Geometry check sheet. Reference: the model listing, model coordinates, mm. A direction names the side the tool comes from. Round coordinates to 2 decimals unless told otherwise and drop trailing zeros. Write each loop counter-clockwise with the first axis right and the second up, starting at its lowest first coordinate (ties: lowest second). Pieces come first, ordered by that corner, then holes. Notation, with made-up numbers: (-29, -29.5) -> (-7, -29.5) arc R33 cw to (-7, 7.5) -> close; hole circle Ø10 at (77.5, 42.5). An arc over 180 degrees is marked (long way). One line per question, with ' | ' between items.
```python
from build123d import *

# Parameters (mm, degrees)
SKETCH1_R           = 1.600003175
SKETCH1_W           = 1.5
SKETCH1_H           = 42.00008382
SKETCH1_W_2         = 92.00018542
SKETCH1_H_2         = 1.5
BOSS_EXTRUDE1_DEPTH = 3
SKETCH1_3_W         = 92.00018542
SKETCH1_3_H         = 1.5
SKETCH1_3_W_2       = 1.5
SKETCH1_3_H_2       = 42.00008382
BOSS_EXTRUDE2_DEPTH = 16


with BuildPart() as part:
    # Sketch1 → Boss-Extrude1 (new body)
    # profile 1 of 17: a face of its own
    with BuildSketch(Plane(origin=(0, 0, 0), x_dir=(1, 0, 0), z_dir=(0, 1, 0))):
        with BuildLine():
            Line((96.00019304, 49.987399035), (4.00000762, 49.987399035))
            ThreePointArc((4.00000762, 49.987399035), (1.180555381, 48.819543679), (0.012700025, 46.00009144))
            Line((0.012700025, 46.00009144), (0.012700025, 4.00000762))
            ThreePointArc((0.012700025, 4.00000762), (1.180555381, 1.180555381), (4.00000762, 0.012700025))
            Line((4.00000762, 0.012700025), (96.00019304, 0.012700025))
            ThreePointArc((96.00019304, 0.012700025), (98.819645279, 1.180555381), (99.987500635, 4.00000762))
            Line((99.987500635, 4.00000762), (99.987500635, 46.00009144))
            ThreePointArc((99.987500635, 46.00009144), (98.819645279, 48.819543679), (96.00019304, 49.987399035))
        make_face()
        with Locations(Location((5.00001016, 45.0000889, 0), (0, 0, 270))):
            Circle(SKETCH1_R, mode=Mode.SUBTRACT)
        with Locations(Location((5.00001016, 5.00001016, 0), (0, 0, 270))):
            Circle(SKETCH1_R, mode=Mode.SUBTRACT)
        with Locations(Location((95.0001905, 5.00001016, 0), (0, 0, 270))):
            Circle(SKETCH1_R, mode=Mode.SUBTRACT)
        with Locations(Location((95.0001905, 45.0000889, 0), (0, 0, 270))):
            Circle(SKETCH1_R, mode=Mode.SUBTRACT)
        with BuildLine():
            Line((85.627156504, 17.327051436), (70.827156816, 17.327051436))
            ThreePointArc((70.827156816, 17.327051436), (70.473603433, 17.473498042), (70.327156827, 17.827051425))
            Line((70.327156827, 17.827051425), (70.327156827, 36.027051041))
            ThreePointArc((70.327156827, 36.027051041), (70.473603433, 36.380604424), (70.827156816, 36.52705103))
            Line((70.827156816, 36.52705103), (85.627156504, 36.52705103))
            ThreePointArc((85.627156504, 36.52705103), (85.980709887, 36.380604424), (86.127156493, 36.027051041))
            Line((86.127156493, 36.027051041), (86.127156493, 17.827051425))
            ThreePointArc((86.127156493, 17.827051425), (85.980709887, 17.473498042), (85.627156504, 17.327051436))
        make_face(mode=Mode.SUBTRACT)
    # profile 2 of 17: a face of its own
    with BuildSketch(Plane(origin=(0, 0, 0), x_dir=(1, 0, 0), z_dir=(0, 1, 0))):
        with Locations((-0.737299975, 25.00004953)):
            Rectangle(SKETCH1_W, SKETCH1_H)
    # profile 3 of 17: a face of its own
    with BuildSketch(Plane(origin=(0, 0, 0), x_dir=(1, 0, 0), z_dir=(0, 1, 0))):
        with Locations((-2.237299975, 25.00004953)):
            Rectangle(SKETCH1_W, SKETCH1_H)
    # profile 4 of 17: a face of its own
    with BuildSketch(Plane(origin=(0, 0, 0), x_dir=(1, 0, 0), z_dir=(0, 1, 0))):
        with BuildLine():
            ThreePointArc((4.00000762, -1.487299975), (0.119895209, 0.119895209), (-1.487299975, 4.00000762))
            Line((-1.487299975, 4.00000762), (-2.987299975, 4.00000762))
            ThreePointArc((-2.987299975, 4.00000762), (-0.940764962, -0.940764962), (4.00000762, -2.987299975))
            Line((4.00000762, -2.987299975), (4.00000762, -1.487299975))
        make_face()
    # profile 5 of 17: a face of its own
    with BuildSketch(Plane(origin=(0, 0, 0), x_dir=(1, 0, 0), z_dir=(0, 1, 0))):
        with BuildLine():
            ThreePointArc((4.00000762, 0.012700025), (1.180555381, 1.180555381), (0.012700025, 4.00000762))
            Line((0.012700025, 4.00000762), (-1.487299975, 4.00000762))
            ThreePointArc((-1.487299975, 4.00000762), (0.119895209, 0.119895209), (4.00000762, -1.487299975))
            Line((4.00000762, -1.487299975), (4.00000762, 0.012700025))
        make_face()
    # profile 6 of 17: a face of its own
    with BuildSketch(Plane(origin=(0, 0, 0), x_dir=(1, 0, 0), z_dir=(0, 1, 0))):
        with Locations((50.00010033, -0.737299975)):
            Rectangle(SKETCH1_W_2, SKETCH1_H_2)
    # profile 7 of 17: a face of its own
    with BuildSketch(Plane(origin=(0, 0, 0), x_dir=(1, 0, 0), z_dir=(0, 1, 0))):
        with Locations((50.00010033, -2.237299975)):
            Rectangle(SKETCH1_W_2, SKETCH1_H_2)
    # profile 8 of 17: a face of its own
    with BuildSketch(Plane(origin=(0, 0, 0), x_dir=(1, 0, 0), z_dir=(0, 1, 0))):
        with BuildLine():
            Line((101.487500635, 4.00000762), (99.987500635, 4.00000762))
            ThreePointArc((99.987500635, 4.00000762), (98.819645279, 1.180555381), (96.00019304, 0.012700025))
            Line((96.00019304, 0.012700025), (96.00019304, -1.487299975))
            ThreePointArc((96.00019304, -1.487299975), (99.880305451, 0.119895209), (101.487500635, 4.00000762))
        make_face()
    # profile 9 of 17: a face of its own
    with BuildSketch(Plane(origin=(0, 0, 0), x_dir=(1, 0, 0), z_dir=(0, 1, 0))):
        with BuildLine():
            Line((102.987500635, 4.00000762), (101.487500635, 4.00000762))
            ThreePointArc((101.487500635, 4.00000762), (99.880305451, 0.119895209), (96.00019304, -1.487299975))
            Line((96.00019304, -1.487299975), (96.00019304, -2.987299975))
            ThreePointArc((96.00019304, -2.987299975), (100.940965623, -0.940764962), (102.987500635, 4.00000762))
        make_face()
    # profile 10 of 17: a face of its own
    with BuildSketch(Plane(origin=(0, 0, 0), x_dir=(1, 0, 0), z_dir=(0, 1, 0))):
        with Locations((100.737500635, 25.00004953)):
            Rectangle(SKETCH1_W, SKETCH1_H)
    # profile 11 of 17: a face of its own
    with BuildSketch(Plane(origin=(0, 0, 0), x_dir=(1, 0, 0), z_dir=(0, 1, 0))):
        with Locations((102.237500635, 25.00004953)):
            Rectangle(SKETCH1_W, SKETCH1_H)
    # profile 12 of 17: a face of its own
    with BuildSketch(Plane(origin=(0, 0, 0), x_dir=(1, 0, 0), z_dir=(0, 1, 0))):
        with BuildLine():
            Line((96.00019304, 51.487399035), (96.00019304, 49.987399035))
            ThreePointArc((96.00019304, 49.987399035), (98.819645279, 48.819543679), (99.987500635, 46.00009144))
            Line((99.987500635, 46.00009144), (101.487500635, 46.00009144))
            ThreePointArc((101.487500635, 46.00009144), (99.880305451, 49.880203851), (96.00019304, 51.487399035))
        make_face()
    # profile 13 of 17: a face of its own
    with BuildSketch(Plane(origin=(0, 0, 0), x_dir=(1, 0, 0), z_dir=(0, 1, 0))):
        with BuildLine():
            Line((96.00019304, 52.987399035), (96.00019304, 51.487399035))
            ThreePointArc((96.00019304, 51.487399035), (99.880305451, 49.880203851), (101.487500635, 46.00009144))
            Line((101.487500635, 46.00009144), (102.987500635, 46.00009144))
            ThreePointArc((102.987500635, 46.00009144), (100.940965623, 50.940864023), (96.00019304, 52.987399035))
        make_face()
    # profile 14 of 17: a face of its own
    with BuildSketch(Plane(origin=(0, 0, 0), x_dir=(1, 0, 0), z_dir=(0, 1, 0))):
        with Locations((50.00010033, 50.737399035)):
            Rectangle(SKETCH1_W_2, SKETCH1_H_2)
    # profile 15 of 17: a face of its own
    with BuildSketch(Plane(origin=(0, 0, 0), x_dir=(1, 0, 0), z_dir=(0, 1, 0))):
        with Locations((50.00010033, 52.237399035)):
            Rectangle(SKETCH1_W_2, SKETCH1_H_2)
    # profile 16 of 17: a face of its own
    with BuildSketch(Plane(origin=(0, 0, 0), x_dir=(1, 0, 0), z_dir=(0, 1, 0))):
        with BuildLine():
            ThreePointArc((0.012700025, 46.00009144), (1.180555381, 48.819543679), (4.00000762, 49.987399035))
            Line((4.00000762, 49.987399035), (4.00000762, 51.487399035))
            ThreePointArc((4.00000762, 51.487399035), (0.119895209, 49.880203851), (-1.487299975, 46.00009144))
            Line((-1.487299975, 46.00009144), (0.012700025, 46.00009144))
        make_face()
    # profile 17 of 17: a face of its own
    with BuildSketch(Plane(origin=(0, 0, 0), x_dir=(1, 0, 0), z_dir=(0, 1, 0))):
        with BuildLine():
            ThreePointArc((-1.487299975, 46.00009144), (0.119895209, 49.880203851), (4.00000762, 51.487399035))
            Line((4.00000762, 51.487399035), (4.00000762, 52.987399035))
            ThreePointArc((4.00000762, 52.987399035), (-0.940764962, 50.940864023), (-2.987299975, 46.00009144))
            Line((-2.987299975, 46.00009144), (-1.487299975, 46.00009144))
        make_face()
    extrude(amount=BOSS_EXTRUDE1_DEPTH)

    # Sketch1_3 → Boss-Extrude2 (add)
    with BuildSketch(Plane(origin=(0, 0, 0), x_dir=(1, 0, 0), z_dir=(0, 1, 0))):
        with BuildLine():
            ThreePointArc((-1.487299975, 46.00009144), (0.119895209, 49.880203851), (4.00000762, 51.487399035))
            Line((4.00000762, 51.487399035), (4.00000762, 52.987399035))
            ThreePointArc((4.00000762, 52.987399035), (-0.940764962, 50.940864023), (-2.987299975, 46.00009144))
            Line((-2.987299975, 46.00009144), (-1.487299975, 46.00009144))
        make_face()
        with Locations((50.00010033, 52.237399035)):
            Rectangle(SKETCH1_3_W, SKETCH1_3_H)
        with BuildLine():
            Line((96.00019304, 52.987399035), (96.00019304, 51.487399035))
            ThreePointArc((96.00019304, 51.487399035), (99.880305451, 49.880203851), (101.487500635, 46.00009144))
            Line((101.487500635, 46.00009144), (102.987500635, 46.00009144))
            ThreePointArc((102.987500635, 46.00009144), (100.940965623, 50.940864023), (96.00019304, 52.987399035))
        make_face()
        with Locations((102.237500635, 25.00004953)):
            Rectangle(SKETCH1_3_W_2, SKETCH1_3_H_2)
        with BuildLine():
            Line((102.987500635, 4.00000762), (101.487500635, 4.00000762))
            ThreePointArc((101.487500635, 4.00000762), (99.880305451, 0.119895209), (96.00019304, -1.487299975))
            Line((96.00019304, -1.487299975), (96.00019304, -2.987299975))
            ThreePointArc((96.00019304, -2.987299975), (100.940965623, -0.940764962), (102.987500635, 4.00000762))
        make_face()
        with Locations((50.00010033, -2.237299975)):
            Rectangle(SKETCH1_3_W, SKETCH1_3_H)
        with BuildLine():
            ThreePointArc((4.00000762, -1.487299975), (0.119895209, 0.119895209), (-1.487299975, 4.00000762))
            Line((-1.487299975, 4.00000762), (-2.987299975, 4.00000762))
            ThreePointArc((-2.987299975, 4.00000762), (-0.940764962, -0.940764962), (4.00000762, -2.987299975))
            Line((4.00000762, -2.987299975), (4.00000762, -1.487299975))
        make_face()
        with Locations((-2.237299975, 25.00004953)):
            Rectangle(SKETCH1_3_W_2, SKETCH1_3_H_2)
    extrude(amount=BOSS_EXTRUDE2_DEPTH)


solid = part.part
```
(1) Draft check along X on faces 1 (the cylindrical face through (5.07, 1.48, -46.6)), 2 (the cylindrical face through (100.89, 7.89, 0.99)), 3 (the cylindrical face through (-0.89, 7.89, -50.99)). Enter one of: +X half, -X half, draft (parallel to the pull), parting line (faces both ways), or undercut.
Resolved:
face 1: undercut | face 2: +X half | face 3: -X half
(2) Sectioned sample at D-D on y = 15. Record the cut outline in (x, z), then the cut area to 3 significant figures.
Resolved:
outline: (-2.99, -46) arc R6.99 ccw to (4, -52.99) -> (96, -52.99) arc R6.99 ccw to (102.99, -46) -> (102.99, -4) arc R6.99 ccw to (96, 2.99) -> (4, 2.99) arc R6.99 ccw to (-2.99, -4) -> close; hole (-1.49, -46) arc R5.49 ccw to (4, -51.49) -> (96, -51.49) arc R5.49 ccw to (101.49, -46) -> (101.49, -4) arc R5.49 ccw to (96, 1.49) -> (4, 1.49) arc R5.49 ccw to (-1.49, -4) -> close | area: 461 mm2
(3) Sectioned sample at C-C on y = 1.25. Record the cut outline in (x, z).
Resolved:
outline: (-2.99, -46) arc R6.99 ccw to (4, -52.99) -> (96, -52.99) arc R6.99 ccw to (102.99, -46) -> (102.99, -4) arc R6.99 ccw to (96, 2.99) -> (4, 2.99) arc R6.99 ccw to (-2.99, -4) -> close; hole circle Ø3.2 at (5, -45); hole circle Ø3.2 at (5, -5); hole (70.33, -36.03) arc R0.5 ccw to (70.83, -36.53) -> (85.63, -36.53) arc R0.5 ccw to (86.13, -36.03) -> (86.13, -17.83) arc R0.5 ccw to (85.63, -17.33) -> (70.83, -17.33) arc R0.5 ccw to (70.33, -17.83) -> close; hole circle Ø3.2 at (95, -45); hole circle Ø3.2 at (95, -5)
(4) Sectioned sample at A-A on z = -19. Record the cut outline in (x, y), then the cut area to 3 significant figures.
Resolved:
outline: (-2.99, 0) -> (70.33, 0) -> (70.33, 3) -> (-1.49, 3) -> (-1.49, 16) -> (-2.99, 16) -> close; (86.13, 0) -> (102.99, 0) -> (102.99, 16) -> (101.49, 16) -> (101.49, 3) -> (86.13, 3) -> close | area: 310 mm2
(5) Material ranges on line 1 (Z direction, x = 22.5, y = 7.5); line 2 (X direction, y = 15, z = -27); line 3 (X direction, y = 1.25, z = -18.5), recorded low to high.
Resolved:
line 1: z = -52.99 to -51.49, 1.49 to 2.99 | line 2: x = -2.99 to -1.49, 101.49 to 102.99 | line 3: x = -2.99 to 70.33, 86.13 to 102.99
(6) Sectioned sample at B-B on x = 74. Record the cut outline in (y, z).
Resolved:
outline: (0, -52.99) -> (16, -52.99) -> (16, -51.49) -> (3, -51.49) -> (3, -36.53) -> (0, -36.53) -> close; (0, -17.33) -> (3, -17.33) -> (3, 1.49) -> (16, 1.49) -> (16, 2.99) -> (0, 2.99) -> close
(7) Go/stop test with flat-tipped pins: pin 1 (16 mm diameter, centred on x = 47.5, z = -25.5, fed in from +Y); pin 2 (2.5 mm diameter, centred on x = 95, z = -45, fed in from -Y). Record where each tip stops, or that it passes through.
Resolved:
pin 1: stops at y = 3 | pin 2: passes through
(8) Access from +Z, -Z, +X, -X, +Y, -Y to the whole of each face (thin tool, end or side, straight path). Record for faces 4 (the flat face through (-2.987, 8, -25)), 5 (the cylindrical face through (0.16, 9.41, -0.08)), 6 (the flat face through (86.127, 1, -27)).
Resolved:
face 4: +Z, -Z, -X, +Y, -Y | face 5: +Y | face 6: +Y, -Y
